from build123d import *

# Parameters (mm, degrees)
F1_DEPTH  = 10
F3_DEPTH  = 10
F5_DEPTH  = 10
F6_R      = 10
F7_DEPTH  = 10.001
F8_R      = 17
F8_R_2    = 10
F9_DEPTH  = 3
F10_R     = 7.5
F11_DEPTH = 58.4585131106


with BuildPart() as f1:
    # F0 (on Top) → F1 (new body)
    with BuildSketch(Plane.XY):
        with BuildLine():
            Line((-29.2287565553, 15), (-29.2287565553, -15))
            Line((-29.2287565553, -15), (-13.2287565553, -15))
            ThreePointArc((-13.2287565553, -15), (0, -20), (13.2287565553, -15))
            Line((13.2287565553, -15), (29.2287565553, -15))
            Line((29.2287565553, -15), (29.2287565553, 15))
            Line((29.2287565553, 15), (13.2287565553, 15))
            ThreePointArc((13.2287565553, 15), (0, 20), (-13.2287565553, 15))
            Line((-13.2287565553, 15), (-29.2287565553, 15))
        make_face()
    extrude(amount=F1_DEPTH)

    # F2 (on face) → F3 (join)
    with BuildSketch(Plane.YZ.offset(29.2287565553)):
        with BuildLine():
            Line((-15, 35), (-15, 10))
            Line((-15, 10), (15, 10))
            Line((15, 10), (15, 35))
            ThreePointArc((15, 35), (0, 50), (-15, 35))
        make_face()
    extrude(amount=-F3_DEPTH)

    # F4 (on face) → F5 (join)
    with BuildSketch(Plane(origin=(-29.2287565553, 0, 0), x_dir=(0, -1, 0), z_dir=(-1, 0, 0))):
        with BuildLine():
            Line((-15, 35), (-15, 10))
            Line((-15, 10), (15, 10))
            Line((15, 10), (15, 35))
            ThreePointArc((15, 35), (0, 50), (-15, 35))
        make_face()
    extrude(amount=-F5_DEPTH)

    # F6 (on face) → F7 (cut, through all)
    with BuildSketch(Plane.XY.offset(10)):
        Circle(F6_R)
    extrude(amount=-F7_DEPTH, mode=Mode.SUBTRACT)

    # F8 (on face) → F9 (join)
    with BuildSketch(Plane(origin=(0, 0, 0), x_dir=(1, 0, 0), z_dir=(0, 0, -1))):
        Circle(F8_R)
        Circle(F8_R_2, mode=Mode.SUBTRACT)
    extrude(amount=F9_DEPTH)

    # F10 (on face) → F11 (cut, through all)
    with BuildSketch(Plane.YZ.offset(29.2287565553)):
        with Locations((0, 35)):
            Circle(F10_R)
    extrude(amount=-F11_DEPTH, mode=Mode.SUBTRACT)


solid = f1.part
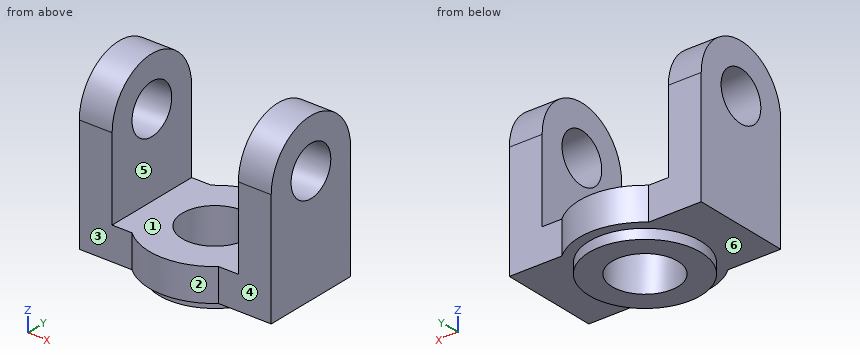
CAD build for the part. Positions are in the model's coordinates, mm. Face numbers are marked on the shaded views. A direction names the side the tool comes from. Give positions to 0.01 mm unless a question says otherwise; leave off trailing zeros. Loops run counter-clockwise (first coordinate to the right, second up) from the corner with the lowest first, then second, coordinate; pieces in that order, holes last. Notation, with made-up numbers: M 20,-1.5 L 42,-1.5 A19 cw 42,9.5 Z; hole C 51,-21.75 d9. An arc over 180 degrees is marked long. Answer in a Markdown table with one row per item. Add a question column.
Item 1: Mould opens along X. For the marked faces 1, 2 and 3 say: +X half, -X half, draft (parallel to the pull), parting line (faces both ways), or undercut.
Item 2: Probe probe 1 along Z at (x, y) = (23, 0); probe 2 along X at (y, z) = (10, 24.5); probe 3 along Y at (x, z) = (0.5, 2). List the from-to ranges inside material, lowest first.
Item 3: Drop flat-ended pins along their axis: P1, Ø10, axis at x = -17.5, z = 26, coming from the +Y side; P2, Ø5, axis at x = 24, z = 23, coming from the -Y side. Give the stop position or say it passes through.
Item 4: Tool access for the marked faces 4, 5 and 6: list every direction of +Z, -Z, +X, -X, +Y, -Y with a clear straight run to the whole face (end or side of a thin tool).
Item 5: Band-saw the part on C-C on y = 0. Give the cut face in (x, z), then the cut area to 3 significant figures.
Item 6: Band-saw the part on B-B on z = 22. Give the cut face in (x, y), then the cut area to 3 significant figures.
Item 7: Band-saw the part on D-D on y = -14. Give the cut face in (x, z), then the cut area to 3 significant figures.
Item 8: Band-saw the part on A-A on x = 0. Give the cut face in (y, z).
Reply:
| question | item | result |
|---|---|---|
| 1 | face 1 | undercut |
| 1 | face 2 | parting line |
| 1 | face 3 | draft |
| 2 | probe 1 | z = 0 to 27.5, 42.5 to 50 |
| 2 | probe 2 | x = -29.23 to -19.23, 19.23 to 29.23 |
| 2 | probe 3 | y = -19.99 to -9.99, 9.99 to 19.99 |
| 3 | P1 | stops at y = 15 |
| 3 | P2 | stops at y = -15 |
| 4 | face 4 | +Z, -Z, +X, -Y |
| 4 | face 5 | +Z, +Y, -Y |
| 4 | face 6 | -Z |
| 5 | outline | M -29.23,0 L -17,0 L -17,-3 L -10,-3 L -10,10 L -19.23,10 L -19.23,27.5 L -29.23,27.5 Z; M -29.23,42.5 L -19.23,42.5 L -19.23,50 L -29.23,50 Z; M 10,-3 L 17,-3 L 17,0 L 29.23,0 L 29.23,27.5 L 19.23,27.5 L 19.23,10 L 10,10 Z; M 19.23,42.5 L 29.23,42.5 L 29.23,50 L 19.23,50 Z |
| 5 | area | 927 mm^2 |
| 6 | outline | M -29.23,-15 L -19.23,-15 L -19.23,15 L -29.23,15 Z; M 19.23,-15 L 29.23,-15 L 29.23,15 L 19.23,15 Z |
| 6 | area | 600 mm^2 |
| 7 | outline | M -29.23,0 L -9.64,0 L -9.64,-3 L 9.64,-3 L 9.64,0 L 29.23,0 L 29.23,40.39 L 19.23,40.39 L 19.23,10 L -19.23,10 L -19.23,40.39 L -29.23,40.39 Z |
| 7 | area | 1,250 mm^2 |
| 8 | outline | M -20,0 L -17,0 L -17,-3 L -10,-3 L -10,10 L -20,10 Z; M 10,-3 L 17,-3 L 17,0 L 20,0 L 20,10 L 10,10 Z |
